CAD build for the part. Positions are in the model's coordinates, mm. Give positions to 0.01 mm unless a question says otherwise; leave off trailing zeros. Loops run counter-clockwise (first coordinate to the right, second up) from the corner with the lowest first, then second, coordinate; pieces in that order, holes last. Notation, with made-up numbers: (-8, 48.25) - (51, 48.25) arc R30 cw to (51, 83.25) - close; hole circle Ø2 at (-25, -17). An arc over 180 degrees is marked (long way). Return JSON: item names as keys, results as strings.
from build123d import *

# Parameters (mm, degrees)
F0_W           = 25.4
F0_H           = 63.5
F1_DEPTH       = 19.05
F1_FACE_W      = 63.5
F1_FACE_H      = 19.05
F3_W           = 63.5
F3_H           = 6.35
F5_D           = 38.1
F8_D           = 6.7564
F8_CSINK_D     = 12.7
F8_CSINK_ANGLE = 82


with BuildPart() as f1:
    # F0 (on Top) → F1 (new body)
    with BuildSketch(Plane.XY):
        with Locations((12.7, 31.75)):
            Rectangle(F0_W, F0_H)
    extrude(amount=F1_DEPTH)

    # F1_face (on face) → F4 section 0
    with BuildSketch(Plane(origin=(25.4, 31.75, 9.525), x_dir=(0, 1, 0), z_dir=(1, 0, 0))):
        Rectangle(F1_FACE_W, F1_FACE_H)
    # F3 (on offset) → F4 section 1
    with BuildSketch(Plane.YZ.offset(50.8)):
        with Locations((31.75, 3.175)):
            Rectangle(F3_W, F3_H)
    loft()

    # F5 (through all)
    with Locations(Plane(origin=(0, 0, 0), x_dir=(1, 0, 0), z_dir=(0, 0, -1))):
        with Locations((50.8, -31.75)):
            Hole(F5_D / 2)

    # F8 (through all)
    with Locations(Plane.XY.offset(19.05)):
        with Locations((12.7, 52.07), (12.7, 31.75), (12.7, 11.43)):
            CounterSinkHole(F8_D / 2, F8_CSINK_D / 2, counter_sink_angle=F8_CSINK_ANGLE)


solid = f1.part
1. Cut at B-B, the plane x = 12.7. Write the cut outline in (y, z), plus the area to 3 significant figures.
Values follow:
{"outline": "(0, 0) - (8.05, 0) - (8.05, 15.63) - (5.08, 19.05) - (0, 19.05) - close; (14.81, 0) - (28.37, 0) - (28.37, 15.63) - (25.4, 19.05) - (17.78, 19.05) - (14.81, 15.63) - close; (35.13, 0) - (48.69, 0) - (48.69, 15.63) - (45.72, 19.05) - (38.1, 19.05) - (35.13, 15.63) - close; (55.45, 0) - (63.5, 0) - (63.5, 19.05) - (58.42, 19.05) - (55.45, 15.63) - close", "area": "793 mm²"}
2. Drop flat-ended pins along their axis: P1, Ø8, axis at x = 12.7, y = 11.43, coming from the +Z side; P2, Ø11, axis at x = 12.7, y = 31.75, coming from the +Z side. Give the stop position or say it passes through.
Values follow:
{"P1": "stops at z = 16.35", "P2": "stops at z = 18.07"}
3. Drill centre lines: probe 1 along Y at (x, z) = (12.7, 7.5); probe 2 along X at (y, z) = (52.07, 5.75); probe 3 along X at (y, z) = (31.75, 9). Where is each one in solid material? Low to high.
Values follow:
{"probe 1": "y = 0 to 8.05, 14.81 to 28.37, 35.13 to 48.69, 55.45 to 63.5", "probe 2": "x = 0 to 9.32, 16.08 to 50.8", "probe 3": "x = 0 to 9.32, 16.08 to 31.75"}
4. Cut at A-A, the plane y = 11.43. Write the cut outline in (x, z), plus the area to 3 significant figures.
Values follow:
{"outline": "(0, 0) - (9.32, 0) - (9.32, 15.63) - (6.35, 19.05) - (0, 19.05) - close; (16.08, 0) - (50.8, 0) - (50.8, 6.35) - (25.4, 19.05) - (19.05, 19.05) - (16.08, 15.63) - close", "area": "668 mm²"}
5. Pull direction X, two halves, no side cores. Call faces 1 (the face through (25, 0, 9)), 2 (the face through (13.46, 28.31, 15.8)), 3 (the face through (0, 31, 9)): +X half, -X half, draft (parallel to the pull), parting line (faces both ways), or undercut.
Values follow:
{"face 1": "draft", "face 2": "undercut", "face 3": "-X half"}
6. Cut at C-C, the plane z = 5. Write the cut outline in (x, y), plus the area to 3 significant figures.
Values follow:
{"outline": "(0, 0) - (50.8, 0) - (50.8, 12.7) arc R19.05 cw to (50.8, 50.8) - (50.8, 63.5) - (0, 63.5) - close; hole circle Ø6.76 at (12.7, 11.43); hole circle Ø6.76 at (12.7, 31.75); hole circle Ø6.76 at (12.7, 52.07)", "area": "2,550 mm²"}
7. Cut at D-D, the plane y = 31.75. Write the cut outline in (x, z) (3 decimals), plus the area to 3 significant figures.
Values follow:
{"outline": "(0, 0) - (9.322, 0) - (9.322, 15.631) - (6.35, 19.05) - (0, 19.05) - close; (16.078, 0) - (31.75, 0) - (31.75, 15.875) - (25.4, 19.05) - (19.05, 19.05) - (16.078, 15.631) - close", "area": "456 mm²"}
